Can you work these out from the model? Positions are in its coordinate system, mm. A direction names the side the tool comes from. Give positions to 0.01 mm unless a question says otherwise; leave off trailing zeros. Write each loop counter-clockwise with the first axis right and the second up, starting at its lowest first coordinate (ties: lowest second). Pieces come first, ordered by that corner, then holes.
1. Suppose I cut it at C-C (y = 17.5). Please give me the cut outline in (x, z), and give its area (3 significant figures).
2. If I drill on probe 1 along Z at (x, y) = (-4, 19); probe 2 along X at (y, z) = (7, -1.45); probe 3 along X at (y, z) = (7, -0.2), over which ranges is the centre line in solid material (lowest first)?
3. Suppose I cut it at B-B (x = -4.5). Please give me the cut outline in (y, z).
4. Suppose I cut it at A-A (z = -1.6). Please give me the cut outline in (x, y), and give its area (3 significant figures).
5. I'm going to push flat-ended pins straight in: pin 1 (2 mm diameter, centred on x = 2.5, y = 28.5, fed in from -Z); pin 2 (0.8 mm diameter, centred on y = 4, z = -0.5, fed in from -X). Where does each tip first touch, or does it pass through?
6. On a 3-axis mill with a long thin cutter (end or side, diameter ignored), from which of +Z, -Z, +X, -X, +Y, -Y can I reach the whole of each face in a straight line? I mean faces 1 (the cylindrical face through (-2.199, 0.285, -0.507)), 2 (the cylindrical face through (2.199, 0.285, -0.507)), 3 (the cylindrical face through (-2.199, 7.215, -0.507)), 4 (the flat face through (0, 7.5, -0.5)). Say none if no direction works.
```python
from build123d import *

# Parameters (mm, degrees)
SKETCH1_W           = 20
SKETCH1_H           = 32.5
BOSS_EXTRUDE1_DEPTH = 2.5
SKETCH2_W           = 5
SKETCH2_H           = 7.5
BOSS_EXTRUDE2_DEPTH = 2
FILLET1_R           = 1


with BuildPart() as part:
    # Sketch1 → Boss-Extrude1 (new body)
    with BuildSketch(Plane.XY):
        with Locations((0, 16.25)):
            Rectangle(SKETCH1_W, SKETCH1_H)
    extrude(amount=BOSS_EXTRUDE1_DEPTH)

    # Sketch2 → Boss-Extrude2 (add)
    with BuildSketch(Plane(origin=(0, 0, 0), x_dir=(-1, 0, 0), z_dir=(0, 0, -1))):
        with Locations((0, 3.75)):
            Rectangle(SKETCH2_W, SKETCH2_H)
    extrude(amount=BOSS_EXTRUDE2_DEPTH)

    # Fillet1
    fillet1_edges = [part.edges().sort_by_distance(p)[0] for p in [
        (2.5, 7.5, -1),
        (2.5, 0, -1),
        (-2.5, 0, -1),
        (-2.5, 7.5, -1),
        (2.5, 3.75, -2),
        (0, 0, -2),
        (-2.5, 3.75, -2),
        (0, 7.5, -2),
    ]]
    fillet(fillet1_edges, radius=FILLET1_R)


solid = part.part
```
Checks:
1. outline: (-10, 0) - (10, 0) - (10, 2.5) - (-10, 2.5) - close
1. area: 50.0 mm2
2. probe 1: z = 0 to 2.5
2. probe 2: x = -2.24 to 2.24
2. probe 3: x = -2.37 to 2.37
3. outline: (0, 0) - (32.5, 0) - (32.5, 2.5) - (0, 2.5) - close
4. outline: (-2.3, 1) arc R0.8 ccw to (-1.5, 0.2) - (1.5, 0.2) arc R0.8 ccw to (2.3, 1) - (2.3, 6.5) arc R0.8 ccw to (1.5, 7.3) - (-1.5, 7.3) arc R0.8 ccw to (-2.3, 6.5) - close
4. area: 32.1 mm2
5. pin 1: stops at z = 0
5. pin 2: stops at x = -2.5
6. face 1: -Z, -X, -Y
6. face 2: -Z, +X, -Y
6. face 3: -Z, -X, +Y
6. face 4: -Z, +X, -X, +Y
